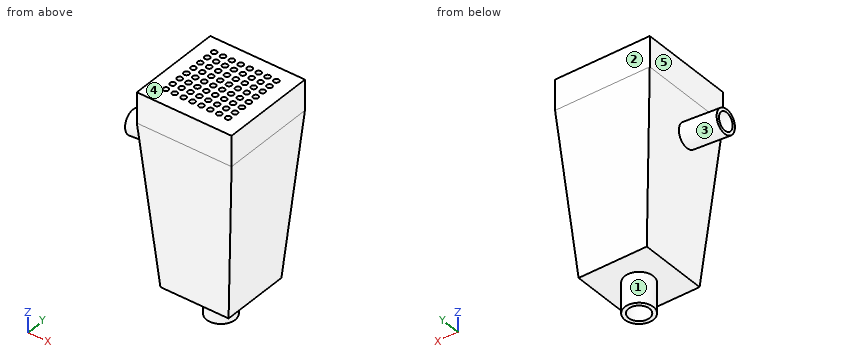
```python
from build123d import *

# Parameters (mm, degrees)
SKETCH2_4_W         = 25
SKETCH2_4_H         = 25
BOSS_EXTRUDE2_DEPTH = 8
SKETCH5_R           = 0.7
CUT_EXTRUDE1_DEPTH  = 8
SKETCH6_R           = 3.1
SKETCH6_R_2         = 2.3
BOSS_EXTRUDE4_DEPTH = 10
CUT_EXTRUDE2_START  = -4
SKETCH6_4_R         = 2.3
CUT_EXTRUDE2_DEPTH  = 4
SKETCH1_7_R         = 3.75
SKETCH1_7_R_2       = 2.75
BOSS_EXTRUDE7_DEPTH = 8


with BuildPart() as part:
    # Sketch1 → Loft1 section 0
    with BuildSketch(Plane.XY):
        with BuildLine():
            Line((-9, 9), (9, 9))
            Line((9, 9), (9, -9))
            Line((9, -9), (-9, -9))
            Line((-9, -9), (-9, 9))
        make_face()
    # Sketch2 → Loft1 section 1
    with BuildSketch(Plane.XY.offset(43)):
        with BuildLine():
            Line((-12.5, 12.5), (12.5, 12.5))
            Line((12.5, 12.5), (12.5, -12.5))
            Line((12.5, -12.5), (-12.5, -12.5))
            Line((-12.5, -12.5), (-12.5, 12.5))
        make_face()
    loft()

    # Cut-Loft1: read off the stored shape, not the designer's step
    # Cut-Loft1: loft between two sections, ruled curve by curve
    cut_loft1_from = [
        Edge.make_bspline([(-1.944543648, -1.944543648, 0), (-1.715376982, -2.173710315, 0), (-1.426368467, -2.37918614, 0), (-0.758106945, -2.668394189, 0), (-0.379695766, -2.75, 0), (0.379695766, -2.75, 0), (0.758106945, -2.668394189, 0), (1.426368467, -2.37918614, 0), (1.715376982, -2.173710315, 0), (1.944543648, -1.944543648, 0)], [0, 0, 0, 0, 0.25, 0.25, 0.5, 0.5, 0.75, 0.75, 1, 1, 1, 1], 3),
        Edge.make_bspline([(1.944543648, -1.944543648, 0), (2.173710315, -1.715376982, 0), (2.37918614, -1.426368467, 0), (2.668394189, -0.758106945, 0), (2.75, -0.379695766, 0), (2.75, 0.379695766, 0), (2.668394189, 0.758106945, 0), (2.37918614, 1.426368467, 0), (2.173710315, 1.715376982, 0), (1.944543648, 1.944543648, 0)], [0, 0, 0, 0, 0.25, 0.25, 0.5, 0.5, 0.75, 0.75, 1, 1, 1, 1], 3),
        Edge.make_bspline([(-1.944543648, 1.944543648, 0), (-2.173710315, 1.715376982, 0), (-2.37918614, 1.426368467, 0), (-2.668394189, 0.758106945, 0), (-2.75, 0.379695766, 0), (-2.75, -0.379695766, 0), (-2.668394189, -0.758106945, 0), (-2.37918614, -1.426368467, 0), (-2.173710315, -1.715376982, 0), (-1.944543648, -1.944543648, 0)], [0, 0, 0, 0, 0.25, 0.25, 0.5, 0.5, 0.75, 0.75, 1, 1, 1, 1], 3),
        Edge.make_bspline([(1.944543648, 1.944543648, 0), (1.715376982, 2.173710315, 0), (1.426368467, 2.37918614, 0), (0.758106945, 2.668394189, 0), (0.379695766, 2.75, 0), (-0.379695766, 2.75, 0), (-0.758106945, 2.668394189, 0), (-1.426368467, 2.37918614, 0), (-1.715376982, 2.173710315, 0), (-1.944543648, 1.944543648, 0)], [0, 0, 0, 0, 0.25, 0.25, 0.5, 0.5, 0.75, 0.75, 1, 1, 1, 1], 3),
    ]
    cut_loft1_to = [
        Edge.make_bspline([(-10, -10, 43), (-8.333333333, -10, 43), (-6.666666667, -10, 43), (-3.333333333, -10, 43), (-1.666666667, -10, 43), (1.666666667, -10, 43), (3.333333333, -10, 43), (6.666666667, -10, 43), (8.333333333, -10, 43), (10, -10, 43)], [0, 0, 0, 0, 0.25, 0.25, 0.5, 0.5, 0.75, 0.75, 1, 1, 1, 1], 3),
        Edge.make_bspline([(10, -10, 43), (10, -8.333333333, 43), (10, -6.666666667, 43), (10, -3.333333333, 43), (10, -1.666666667, 43), (10, 1.666666667, 43), (10, 3.333333333, 43), (10, 6.666666667, 43), (10, 8.333333333, 43), (10, 10, 43)], [0, 0, 0, 0, 0.25, 0.25, 0.5, 0.5, 0.75, 0.75, 1, 1, 1, 1], 3),
        Edge.make_bspline([(-10, 10, 43), (-10, 8.333333333, 43), (-10, 6.666666667, 43), (-10, 3.333333333, 43), (-10, 1.666666667, 43), (-10, -1.666666667, 43), (-10, -3.333333333, 43), (-10, -6.666666667, 43), (-10, -8.333333333, 43), (-10, -10, 43)], [0, 0, 0, 0, 0.25, 0.25, 0.5, 0.5, 0.75, 0.75, 1, 1, 1, 1], 3),
        Edge.make_bspline([(10, 10, 43), (8.333333333, 10, 43), (6.666666667, 10, 43), (3.333333333, 10, 43), (1.666666667, 10, 43), (-1.666666667, 10, 43), (-3.333333333, 10, 43), (-6.666666667, 10, 43), (-8.333333333, 10, 43), (-10, 10, 43)], [0, 0, 0, 0, 0.25, 0.25, 0.5, 0.5, 0.75, 0.75, 1, 1, 1, 1], 3),
    ]
    cut_loft1 = Solid(Shell([*[Face.make_surface_from_curves(cut_loft1_from[k], cut_loft1_to[k]) for k in range(4)], Face(Wire(cut_loft1_from)), Face(Wire(cut_loft1_to))]))
    add(cut_loft1, mode=Mode.SUBTRACT)

    # Sketch2<4> → Boss-Extrude2 (add)
    with BuildSketch(Plane.XY.offset(43)):
        Rectangle(SKETCH2_4_W, SKETCH2_4_H)
    extrude(amount=BOSS_EXTRUDE2_DEPTH)

    # Sketch5 → Cut-Extrude1 (cut)
    with BuildSketch(Plane.XY.offset(43)):
        with Locations((-8.388056057, 8.509622087)):
            Circle(SKETCH5_R)
        with Locations((-6.038056057, 8.509622087)):
            Circle(SKETCH5_R)
        with Locations((-3.688056057, 8.509622087)):
            Circle(SKETCH5_R)
        with Locations((-1.338056057, 8.509622087)):
            Circle(SKETCH5_R)
        with Locations((1.011943943, 8.509622087)):
            Circle(SKETCH5_R)
        with Locations((3.361943943, 8.509622087)):
            Circle(SKETCH5_R)
        with Locations((5.711943943, 8.509622087)):
            Circle(SKETCH5_R)
        with Locations((8.061943943, 8.509622087)):
            Circle(SKETCH5_R)
        with Locations((-6.038056057, 6.159622087)):
            Circle(SKETCH5_R)
        with Locations((-3.688056057, 6.159622087)):
            Circle(SKETCH5_R)
        with Locations((-1.338056057, 6.159622087)):
            Circle(SKETCH5_R)
        with Locations((1.011943943, 6.159622087)):
            Circle(SKETCH5_R)
        with Locations((3.361943943, 6.159622087)):
            Circle(SKETCH5_R)
        with Locations((5.711943943, 6.159622087)):
            Circle(SKETCH5_R)
        with Locations((8.061943943, 6.159622087)):
            Circle(SKETCH5_R)
        with Locations((-6.038056057, 3.809622087)):
            Circle(SKETCH5_R)
        with Locations((-3.688056057, 3.809622087)):
            Circle(SKETCH5_R)
        with Locations((-1.338056057, 3.809622087)):
            Circle(SKETCH5_R)
        with Locations((1.011943943, 3.809622087)):
            Circle(SKETCH5_R)
        with Locations((3.361943943, 3.809622087)):
            Circle(SKETCH5_R)
        with Locations((5.711943943, 3.809622087)):
            Circle(SKETCH5_R)
        with Locations((8.061943943, 3.809622087)):
            Circle(SKETCH5_R)
        with Locations((-6.038056057, 1.459622087)):
            Circle(SKETCH5_R)
        with Locations((-3.688056057, 1.459622087)):
            Circle(SKETCH5_R)
        with Locations((-1.338056057, 1.459622087)):
            Circle(SKETCH5_R)
        with Locations((1.011943943, 1.459622087)):
            Circle(SKETCH5_R)
        with Locations((3.361943943, 1.459622087)):
            Circle(SKETCH5_R)
        with Locations((5.711943943, 1.459622087)):
            Circle(SKETCH5_R)
        with Locations((8.061943943, 1.459622087)):
            Circle(SKETCH5_R)
        with Locations((-6.038056057, -0.890377913)):
            Circle(SKETCH5_R)
        with Locations((-3.688056057, -0.890377913)):
            Circle(SKETCH5_R)
        with Locations((-1.338056057, -0.890377913)):
            Circle(SKETCH5_R)
        with Locations((1.011943943, -0.890377913)):
            Circle(SKETCH5_R)
        with Locations((3.361943943, -0.890377913)):
            Circle(SKETCH5_R)
        with Locations((5.711943943, -0.890377913)):
            Circle(SKETCH5_R)
        with Locations((8.061943943, -0.890377913)):
            Circle(SKETCH5_R)
        with Locations((-6.038056057, -3.240377913)):
            Circle(SKETCH5_R)
        with Locations((-3.688056057, -3.240377913)):
            Circle(SKETCH5_R)
        with Locations((-1.338056057, -3.240377913)):
            Circle(SKETCH5_R)
        with Locations((1.011943943, -3.240377913)):
            Circle(SKETCH5_R)
        with Locations((3.361943943, -3.240377913)):
            Circle(SKETCH5_R)
        with Locations((5.711943943, -3.240377913)):
            Circle(SKETCH5_R)
        with Locations((8.061943943, -3.240377913)):
            Circle(SKETCH5_R)
        with Locations((-6.038056057, -5.590377913)):
            Circle(SKETCH5_R)
        with Locations((-3.688056057, -5.590377913)):
            Circle(SKETCH5_R)
        with Locations((-1.338056057, -5.590377913)):
            Circle(SKETCH5_R)
        with Locations((1.011943943, -5.590377913)):
            Circle(SKETCH5_R)
        with Locations((3.361943943, -5.590377913)):
            Circle(SKETCH5_R)
        with Locations((5.711943943, -5.590377913)):
            Circle(SKETCH5_R)
        with Locations((8.061943943, -5.590377913)):
            Circle(SKETCH5_R)
        with Locations((-6.038056057, -7.940377913)):
            Circle(SKETCH5_R)
        with Locations((-3.688056057, -7.940377913)):
            Circle(SKETCH5_R)
        with Locations((-1.338056057, -7.940377913)):
            Circle(SKETCH5_R)
        with Locations((1.011943943, -7.940377913)):
            Circle(SKETCH5_R)
        with Locations((3.361943943, -7.940377913)):
            Circle(SKETCH5_R)
        with Locations((5.711943943, -7.940377913)):
            Circle(SKETCH5_R)
        with Locations((8.061943943, -7.940377913)):
            Circle(SKETCH5_R)
        with Locations((-8.388056057, 6.159622087)):
            Circle(SKETCH5_R)
        with Locations((-8.388056057, 3.809622087)):
            Circle(SKETCH5_R)
        with Locations((-8.388056057, 1.459622087)):
            Circle(SKETCH5_R)
        with Locations((-8.388056057, -0.890377913)):
            Circle(SKETCH5_R)
        with Locations((-8.388056057, -3.240377913)):
            Circle(SKETCH5_R)
        with Locations((-8.388056057, -5.590377913)):
            Circle(SKETCH5_R)
        with Locations((-8.388056057, -7.940377913)):
            Circle(SKETCH5_R)
    extrude(amount=CUT_EXTRUDE1_DEPTH, mode=Mode.SUBTRACT)

    # Sketch6 → Boss-Extrude4 (add)
    with BuildSketch(Plane(origin=(-8.940765615, 0, -0.727736736), x_dir=(-0.08112705090276601, 0, 0.9967037682339824), z_dir=(-0.9967037682339824, 0, -0.08112705090276602))):
        with Locations(Location((34.477535136, -1.520969622, 0), (0, 0, 180))):
            Circle(SKETCH6_R)
        with Locations((34.477535136, -1.520969622)):
            Circle(SKETCH6_R_2, mode=Mode.SUBTRACT)
    extrude(amount=BOSS_EXTRUDE4_DEPTH)

    # Sketch6<4> → Cut-Extrude2 (cut)
    with BuildSketch(Plane(origin=(-8.940765615, 0, -0.727736736), x_dir=(-0.08112705090276601, 0, 0.9967037682339824), z_dir=(-0.9967037682339824, 0, -0.08112705090276602)).offset(CUT_EXTRUDE2_START)):
        with Locations((34.477535136, -1.520969622)):
            Circle(SKETCH6_4_R)
    extrude(amount=CUT_EXTRUDE2_DEPTH, mode=Mode.SUBTRACT)

    # Sketch1<7> → Boss-Extrude7 (add)
    with BuildSketch(Plane.XY):
        Circle(SKETCH1_7_R)
        Circle(SKETCH1_7_R_2, mode=Mode.SUBTRACT)
    extrude(amount=-BOSS_EXTRUDE7_DEPTH)


solid = part.part
```
Geometry: final body of the model. Coordinates: model frame, mm. Face numbers are marked on the shaded views. A direction names the side the tool comes from. Round coordinates to 2 decimals unless told otherwise and drop trailing zeros. Write item = value, one per line. Start each with the question number.
Q1. Pin query (flat end, axial travel): pin 1 (0.8 mm diameter, centred on x = 1.01, y = -7.94, fed in from -Z); pin 2 (6 mm diameter, centred on y = 3.5, z = 4, fed in from +X); pin 3 (3 mm diameter, centred on x = -1.5, z = 40.5, fed in from +Y). Return the tip coordinate at first contact, or that it passes through.
Q2. Access query for the marked faces 1 and 2. Directions: +Z, -Z, +X, -X, +Y, -Y. A direction counts if a zero-diameter tool reaches every point of the face in a straight line with its end or side. Return the directions, or none.
Q3. Ray query, line 1 (X direction, y = -6.5, z = 44); line 2 (X direction, y = -0.5, z = 7); line 3 (Y direction, x = -14, z = 31.5). Return the intervals inside material, ascending. Write a range as from..to.
Q4. Pull-direction query (X, two-part tool) for the marked faces 3, 4 and 5; classes: +X half, -X half, draft (parallel to the pull), parting line (faces both ways), or undercut.
Outcome:
q1.pin_1 = 0
q1.pin_2 = 9.57
q1.pin_3 = 12.42
q2.face_1 = -Z
q2.face_2 = +Z, -Z, +X, -X, +Y
q3.line_1 = -12.5..12.5
q3.line_2 = -9.57..-3.91, 3.91..9.57
q3.line_3 = -3.93..-2.75, -0.29..0.89
q4.face_3 = undercut
q4.face_4 = draft
q4.face_5 = -X half
